```python
from build123d import *

# Parameters (mm, degrees)
BOSS_EXTRUDE1_DEPTH        = 22.5
M4X0_7_TAPPED_HOLE2_REACH  = 42.528
M4X0_7_TAPPED_HOLE2_BORE_R = 1.65
FILLET2_R                  = 2
FILLET3_START              = -23
FILLET3_DEPTH              = 46
FILLET4_START              = -22.5
FILLET4_DEPTH              = 45
FILLET5_R                  = 2
FILLET7_R                  = 14
CUT_EXTRUDE5_DEPTH         = 5
FILLET8_R                  = 0.5
M3X0_5_TAPPED_HOLE1_D      = 2.5
M3X0_5_TAPPED_HOLE1_DEPTH  = 5
M3X0_5_TAPPED_HOLE1_TIP    = 0.751075774
SKETCH20_W                 = 4
SKETCH20_H                 = 2
BOSS_EXTRUDE3_DEPTH        = 15


with BuildPart() as part:
    # Sketch1 → Boss-Extrude1 (new, symmetric)
    with BuildSketch(Plane.XY):
        with BuildLine():
            Line((7.142207986, -17.288856719), (7.142207986, -22.696678834))
            ThreePointArc((7.142207986, -22.696678834), (3.836331075, -24.774076114), (0, -25.5))
            Line((0, -25.5), (-12, -25.5))
            Line((-12, -25.5), (-12, 17.849242405))
            Line((-12, 17.849242405), (-7.424621202, 22.424621202))
            ThreePointArc((-7.424621202, 22.424621202), (-4.01817604, 24.700735091), (0, 25.5))
            Line((0, 25.5), (0, 22.5))
            ThreePointArc((0, 22.5), (-7.047694656, 12.434848925), (4.820907073, 9.254666677))
            Line((4.820907073, 9.254666677), (4.820907073, 6))
            Line((4.820907073, 6), (-8, 6))
            Line((-8, 6), (-8, -6))
            Line((-8, -6), (-4, -6))
            Line((-4, -6), (-4, -8.65571123))
            ThreePointArc((-4, -8.65571123), (-4.593600768, -20.928645038), (7.142207986, -17.288856719))
        make_face()
    extrude(amount=BOSS_EXTRUDE1_DEPTH, both=True)

    # M4x0.7 Tapped Hole2 bore → M4x0.7 Tapped Hole2 (cut, up to next)
    with BuildSketch(Plane(origin=(0, 6, 0), x_dir=(-1, 0, 0), z_dir=(0, -1, 0)), mode=Mode.PRIVATE) as m4x0_7_tapped_hole2_sk1:
        with Locations((0, -17.5)):
            Circle(M4X0_7_TAPPED_HOLE2_BORE_R)
    m4x0_7_tapped_hole2_tool1 = extrude(m4x0_7_tapped_hole2_sk1.sketch, amount=-M4X0_7_TAPPED_HOLE2_REACH, mode=Mode.PRIVATE) & part.part
    # M4x0.7 Tapped Hole2 bore → M4x0.7 Tapped Hole2 (cut, up to next)
    with BuildSketch(Plane(origin=(0, 6, 0), x_dir=(-1, 0, 0), z_dir=(0, -1, 0)), mode=Mode.PRIVATE) as m4x0_7_tapped_hole2_sk2:
        with Locations((0, 17.5)):
            Circle(M4X0_7_TAPPED_HOLE2_BORE_R)
    m4x0_7_tapped_hole2_tool2 = extrude(m4x0_7_tapped_hole2_sk2.sketch, amount=-M4X0_7_TAPPED_HOLE2_REACH, mode=Mode.PRIVATE) & part.part
    add(m4x0_7_tapped_hole2_tool1.solids().sort_by_distance((0, 6, 17.5))[0], mode=Mode.SUBTRACT)
    add(m4x0_7_tapped_hole2_tool2.solids().sort_by_distance((0, 6, -17.5))[0], mode=Mode.SUBTRACT)

    # Fillet2
    # the kernel refuses this fillet: 2 mm, written as the material it adds along each edge
    with BuildSketch(Plane(origin=(-8, -6, 22.5), x_dir=(0, 1, 0), z_dir=(0, 0, -1)), Plane(origin=(-8, 6, 22.5), x_dir=(1, 0, 0), z_dir=(0, 0, -1))) as fillet2_piece_1:
        with BuildLine():
            CenterArc((FILLET2_R, FILLET2_R), FILLET2_R, 180, 90)
            Line((0, FILLET2_R), (0, 0))
            Line((0, 0), (FILLET2_R, 0))
        make_face()
    extrude(amount=45)
    # the kernel refuses this fillet: 2 mm, written as the material it takes off along each edge
    with BuildSketch(Plane(origin=(-4, -8.65571123, -25.052927903), x_dir=(-0.8120954257724025, -0.5835246519552882, 0), z_dir=(0, 0, 1))) as fillet2_2_piece_1:
        with BuildLine():
            CenterArc((1.028312305, -1.996337733), FILLET2_R, 93.46787904, 50.833289284)
            Line((-0.595878546, -0.829288429), (0, 0))
            ThreePointArc((0, 0), (0.453667193, -0.013733502), (0.907334387, 0))
        make_face()
    extrude(amount=50.105855806, mode=Mode.SUBTRACT)
    with BuildSketch(Plane(origin=(-4, -6, -27.5), x_dir=(0, -1, 0), z_dir=(0, 0, 1)), Plane(origin=(4.820907073, 6, 27.5), x_dir=(0, 1, 0), z_dir=(0, 0, -1))) as fillet2_2_piece_2:
        with BuildLine():
            CenterArc((FILLET2_R, -FILLET2_R), FILLET2_R, 90, 90)
            Line((0, -FILLET2_R), (0, 0))
            Line((0, 0), (FILLET2_R, 0))
        make_face()
    extrude(amount=55, mode=Mode.SUBTRACT)

    # Fillet3: read off the stored shape, not the designer's step
    # Fillet3 outline → Fillet3 (cut)
    with BuildSketch(Plane.XY.offset(FILLET3_START)):
        with BuildLine():
            ThreePointArc((0, 25.5), (-0.878075733, 25.463220489), (-1.75, 25.35313962))
            add(Edge.make_bspline(
                [(-1.75, 25.35313962), (-1.340626415, 25.422336386), (-0.839763435, 25.364052085), (-0.332775331, 25.08288536), (1e-09, 24.544131647), (0, 23.874119673)],
                knots=[0, 0, 0, 0, 0, 0, 0.541960109, 0.541960109, 0.541960109, 0.541960109, 0.541960109, 0.541960109], degree=5, weights=[1, 0.783215957, 0.625176065, 0.525880325, 0.485328737, 0.503521301]))
            Line((0, 23.874119673), (0, 25.5))
        make_face()
        with BuildLine():
            Line((0, 22.5), (0, 23.874119673))
            add(Edge.make_bspline(
                [(0, 23.874119673), (-1e-09, 23.344488498), (-0.216926345, 22.902050344), (-0.555121167, 22.607049118), (-0.918235372, 22.451178186), (-1.25, 22.395099729)],
                knots=[0.541960109, 0.541960109, 0.541960109, 0.541960109, 0.541960109, 0.541960109, 1, 1, 1, 1, 1, 1], degree=5, weights=[0.503521301, 0.518896824, 0.576232456, 0.675528195, 0.816784043, 1]))
            ThreePointArc((-1.25, 22.395099729), (-0.627196952, 22.473728921), (0, 22.5))
        make_face()
    extrude(amount=FILLET3_DEPTH, mode=Mode.SUBTRACT)

    # Fillet4: read off the stored shape, not the designer's step
    # Fillet4 outline → Fillet4 (cut)
    with BuildSketch(Plane.XY.offset(FILLET4_START)):
        with BuildLine():
            ThreePointArc((7.142207986, -17.288856719), (6.182933262, -19.245154446), (4.701839989, -20.843175568))
            add(Edge.make_bspline(
                [(4.701839989, -20.843175568), (5.135113998, -20.494532089), (5.812281829, -20.26945545), (6.615008937, -20.444697489), (7.14219213, -21.142606567), (7.142207986, -22.011783319)],
                knots=[0, 0, 0, 0, 0, 0, 0.676183816, 0.676183816, 0.676183816, 0.676183816, 0.676183816, 0.676183816], degree=5, weights=[1, 0.729526474, 0.550497858, 0.462914153, 0.466775358, 0.562081474]))
            Line((7.142207986, -22.011783319), (7.142207986, -17.288856719))
        make_face()
        with BuildLine():
            Line((7.142207986, -22.696678834), (7.142207986, -22.011783319))
            add(Edge.make_bspline(
                [(7.142207986, -22.011783319), (7.142213818, -22.331484727), (7.059225631, -22.61727017), (6.921863818, -22.854436912), (6.756468906, -23.040519024), (6.582575984, -23.180445796)],
                knots=[0.676183816, 0.676183816, 0.676183816, 0.676183816, 0.676183816, 0.676183816, 1, 1, 1, 1, 1, 1], degree=5, weights=[0.562081474, 0.607722411, 0.674334732, 0.761918437, 0.870473526, 1]))
            ThreePointArc((6.582575984, -23.180445796), (6.866653579, -22.943492218), (7.142207986, -22.696678834))
        make_face()
    extrude(amount=FILLET4_DEPTH, mode=Mode.SUBTRACT)

    # Fillet5
    # the kernel refuses this fillet: 2 mm, written as the material it takes off along each edge
    with BuildSketch(Plane(origin=(4.820907073, 9.254666677, 27.882265511), x_dir=(-0.8503705465795661, -0.5261843151500908, 0), z_dir=(0, 0, -1))) as fillet5_piece_1:
        with BuildLine():
            CenterArc((2.439960365, -1.97929278), FILLET5_R, 98.251994966, 54.607083408)
            Line((0.660185926, -1.066931588), (0.624590437, -1.048684364))
            ThreePointArc((0.624590437, -1.048684364), (0.296078141, -0.554513166), (-0.034014822, -0.021047373))
            Line((-0.034014822, -0.021047373), (0.005741083, 0.039585856))
            ThreePointArc((0.005741083, 0.039585856), (1.076453102, -0.037652075), (2.147165121, 0.039585856))
            Line((2.147165121, 0.039585856), (2.152906205, 0))
        make_face()
    extrude(amount=55.764531023, mode=Mode.SUBTRACT)

    # Fillet7
    fillet7_edges = [part.edges().sort_by_distance(p)[0] for p in [
        (-12, 17.849242405, 0),
    ]]
    fillet(fillet7_edges, radius=FILLET7_R)

    # Sketch17 → Cut-Extrude5 (cut)
    with BuildSketch(Plane.XZ.offset(25.5)):
        Polygon((-12, 7.5), (-10, 9.5), (-10, -9.5), (-12, -7.5), align=None)
    extrude(amount=-CUT_EXTRUDE5_DEPTH, mode=Mode.SUBTRACT)

    # Fillet8
    fillet8_edges = [part.edges().sort_by_distance(p)[0] for p in [
        (-12, -23, -7.5),
        (-12, -23, 7.5),
        (-10, -23, 9.5),
        (-10, -23, -9.5),
    ]]
    fillet(fillet8_edges, radius=FILLET8_R)

    # M3x0.5 Tapped Hole1
    with Locations(Plane.ZY.offset(12)):
        with Locations((-10, 15.1), (-10, -4.9), (10, -4.9), (10, 15.1)):
            Hole(M3X0_5_TAPPED_HOLE1_D / 2, depth=M3X0_5_TAPPED_HOLE1_DEPTH)
            with Locations((0, 0, -(M3X0_5_TAPPED_HOLE1_DEPTH + M3X0_5_TAPPED_HOLE1_TIP / 2))):  # 118° drill point
                Cone(0, M3X0_5_TAPPED_HOLE1_D / 2, M3X0_5_TAPPED_HOLE1_TIP, mode=Mode.SUBTRACT)

    # Sketch20 → Boss-Extrude3 (add)
    with BuildSketch(Plane(origin=(0, 0, -22.5), x_dir=(-1, 0, 0), z_dir=(0, 0, -1))):
        with Locations((10, 0.5)):
            Rectangle(SKETCH20_W, SKETCH20_H)
    extrude(amount=BOSS_EXTRUDE3_DEPTH)


solid = part.part
```
CAD build for the part. Positions are in the model's coordinates, mm. A direction names the side the tool comes from. Coordinates: 2 decimals unless noted, no trailing zeros. Order: outer loops, then holes, each group sorted by start corner. A loop starts at its lowest first (then second) coordinate and runs counter-clockwise, first axis right, second up. Notation, with made-up numbers: M 28.25,44 L 52.25,44 A13 ccw 52.25,63 Z; hole C -32.75,84.5 d5. An arc over 180 degrees is marked long. Write each question's results on one line, items separated by ' | '. Start each with the question number.
Q1. Pull direction X, two halves, no side cores. Call faces 1 (the cylindrical face through (1.65, 6.83, 17.43)), 2 (the cylindrical face through (-10.964, 17.337, -0.315)), 3 (the cylindrical face through (-9.6, 13.88, -9.73)): +X half, -X half, draft (parallel to the pull), parting line (faces both ways), or undercut.
Q2. Cut at B-B (y = 15.1). List the corners of the cut face in (x, z).
Q3. Cut at A-A (x = 4). List the corners of the cut face in (y, z), then the cut area to 3 significant figures.
Q4. Drill centre lines: probe 1 along Z at (x, y) = (0, 6.65); probe 2 along Z at (x, y) = (-10.85, 15.1); probe 3 along Y at (x, z) = (-6.5, 4). Where is each one in solid material? Low to high. Write a range as from..to.
Q5. Cut at D-D (z = -10). Count the separate pieces of the cut face and the enclosed holes in it, then the cut area to 3 significant figures.
Q6. Which spindle directions (+Z, -Z, +X, -X, +Y, -Y) get a long thin tool onto all of the face, cutting with end or side? Do faces 4 (the flat face through (-10, -0.5, -30)), 5 (the cylindrical face through (1.65, 6.83, -17.57)), 6 (the cylindrical face through (-10.02, -6.12, -9.73)), 7 (the cylindrical face through (3.5, -24.9, 0.3)), 8 (the flat face through (-10, 1.5, -30)). Say none if no direction does.
Q7. Cut at C-C (z = -27). List the corners of the cut face in (x, y).
Q8. Flat gauge pins, fed straight in: P1, Ø1, axis at y = 15.5, z = -16.5, coming from the -X side; P2, Ø2, axis at y = 15.1, z = -10, coming from the -X side; P3, Ø1.2, axis at x = -11, z = -31.5, coming from the +Y side; P4, Ø4.5, axis at x = -10.5, z = -29, coming from the -Y side. Where does each tip first touch, or does it go through?
Found:
1) face 1: undercut | face 2: -X half | face 3: draft
2) outline: M -11.66,-22.5 L -7.5,-22.5 L -7.5,-11.25 L -11.66,-11.25 Z; M -11.66,-8.75 L -7.5,-8.75 L -7.5,8.75 L -11.66,8.75 Z; M -11.66,11.25 L -7.5,11.25 L -7.5,22.5 L -11.66,22.5 Z
3) outline: M -24.71,-22.5 L -21.34,-22.5 L -21.34,22.5 L -24.71,22.5 Z; M 6.38,-22.5 L 8.28,-22.5 L 8.28,22.5 L 6.38,22.5 Z | area: 237 mm²
4) probe 1: -22.5..-19.15, -15.85..15.85, 19.15..22.5 | probe 2: -22.5..-11.25, -8.75..8.75, 11.25..22.5 | probe 3: -25.5..-18.74, -11.26..-5.94, 5.94..11.26, 18.74..23.25
5) separate pieces: 3 | enclosed holes: 0 | area: 304 mm²
6) face 4: -Z, +X, -X, -Y | face 5: none | face 6: -X | face 7: +Z, -Z, +X, -Y | face 8: -Z, +X, -X, +Y
7) outline: M -12,-0.5 L -8,-0.5 L -8,1.5 L -12,1.5 Z
8) P1: x = -11.69 | P2: through | P3: y = 1.5 | P4: y = -0.5
